For this review, use the dimensioned drawing (mm, ordinates from the lowest corner) and the shaded views. A direction names the side the tool comes from. Give positions to 0.01 mm unless a question says otherwise; leave off trailing zeros. Order: outer loops, then holes, each group sorted by start corner. A loop starts at its lowest first (then second) coordinate and runs counter-clockwise, first axis right, second up. Notation, with made-up numbers: (-8, -11) -> (22, -11) arc R22 ccw to (22, 8) -> close; hole circle Ø11 at (-25, 7.5). An arc over 180 degrees is marked (long way). Return JSON: item names as keys, results as strings.
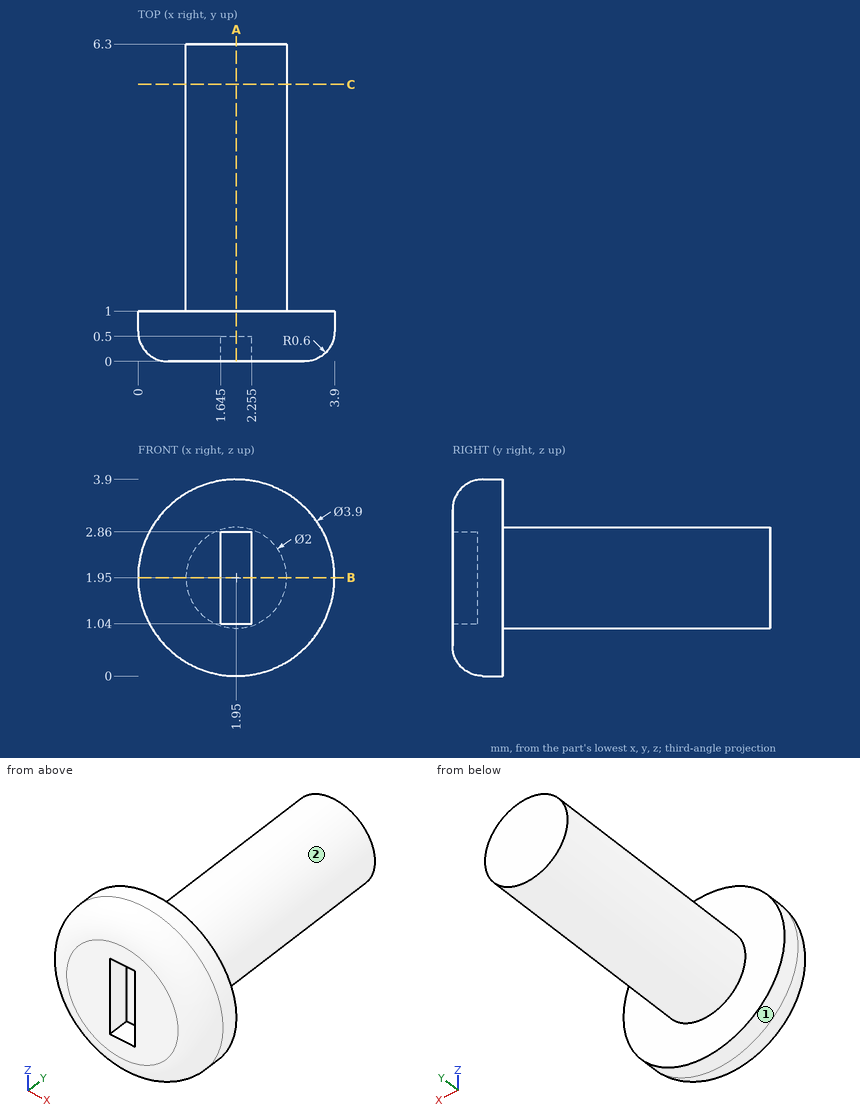
Item 1: Add section B-B (z = 1.95). Give the boundary of the cut face in (x, y) (3 decimals), plus the area to 3 significant figures.
Result set:
{"outline": "(0, 0.6) arc R0.6 ccw to (0.6, 0) -> (1.645, 0) -> (1.645, 0.5) -> (2.255, 0.5) -> (2.255, 0) -> (3.3, 0) arc R0.6 ccw to (3.9, 0.6) -> (3.9, 1) -> (2.95, 1) -> (2.95, 6.3) -> (0.95, 6.3) -> (0.95, 1) -> (0, 1) -> close", "area": "14.0 mm^2"}
Item 2: Machinability: for the marked faces 1 and 2, which of the approach directions +Z, -Z, +X, -X, +Y, -Y give a long, thin tool a straight path to every point of the face, cutting with its end or side? Answer none if there is none.
Result set:
{"face 1": "+Y, -Y", "face 2": "+Y"}
Item 3: Add section A-A (x = 1.95). Give the boundary of the cut face in (y, z).
Result set:
{"outline": "(0, 0.6) arc R0.6 ccw to (0.6, 0) -> (1, 0) -> (1, 0.95) -> (6.3, 0.95) -> (6.3, 2.95) -> (1, 2.95) -> (1, 3.9) -> (0.6, 3.9) arc R0.6 ccw to (0, 3.3) -> (0, 2.86) -> (0.5, 2.86) -> (0.5, 1.04) -> (0, 1.04) -> close"}
Item 4: Wall thickness on L1, parallel to Y at x = 1.7, z = 2.65; L2, parallel to Y at x = 1.9, z = 3.15; L3, parallel to Z at x = 1.9, y = 3: over which ranges is each line inside the solid? List them lowest first. Write a range as [from, to].
Result set:
{"L1": "y = [0.5, 6.3]", "L2": "y = [0, 1]", "L3": "z = [0.95, 2.95]"}
Item 5: For pin 1 (0.6 mm diameter, centred on y = 0.5, z = 1.5, fed in from +X); pin 2 (2 mm diameter, centred on y = 3.5, z = 1, fed in from +X), all flat-tipped, find the tip position at first contact; note any pin that passes through.
Result set:
{"pin 1": "stops at x = 3.89", "pin 2": "stops at x = 2.95"}
Item 6: Add section C-C (y = 5.5). Give the boundary of the cut face in (x, z), plus the area to 3 significant figures.
Result set:
{"outline": "circle Ø2 at (1.95, 1.95)", "area": "3.14 mm^2"}
